from build123d import *

# Parameters (mm, degrees)
SKETCH1_W                   = 33
SKETCH1_H                   = 26
BOSS_EXTRUDE1_DEPTH         = 3.1
SKETCH3_W                   = 4
SKETCH3_H                   = 18
BOSS_EXTRUDE2_DEPTH         = 0.1
TAP_DRILL_FOR_M2X0_4_TAP2_D = 1.8
FILLET2_R                   = 1
SKETCH11_W                  = 21
SKETCH11_H                  = 14
CUT_EXTRUDE2_DEPTH          = 25.459005547


with BuildPart() as part:
    # Sketch1 → Boss-Extrude1 (new body)
    with BuildSketch(Plane(origin=(0, 0, 0), x_dir=(1, 0, 0), z_dir=(0, 1, 0))):
        with Locations((1.816045381, -2.910858995)):
            Rectangle(SKETCH1_W, SKETCH1_H)
    extrude(amount=BOSS_EXTRUDE1_DEPTH)

    # Sketch3 → Boss-Extrude2 (add)
    with BuildSketch(Plane(origin=(0, 3.1, 0), x_dir=(1, 0, 0), z_dir=(0, 1, 0))):
        Polygon((-10.683954619, 10.089141005), (-14.683954619, 10.089141005), (-14.683954619, -15.910858995), (-10.683954619, -15.910858995), (-10.683954619, -11.910858995), (-10.683954619, 6.089141005), align=None)
        Polygon((18.316045381, 10.089141005), (-10.683954619, 10.089141005), (-10.683954619, 6.089141005), (14.316045381, 6.089141005), (18.316045381, 6.089141005), align=None)
        Polygon((-10.683954619, -11.910858995), (-10.683954619, -15.910858995), (18.316045381, -15.910858995), (18.316045381, -11.910858995), (14.316045381, -11.910858995), align=None)
        with Locations((16.316045381, -2.910858995)):
            Rectangle(SKETCH3_W, SKETCH3_H)
    extrude(amount=BOSS_EXTRUDE2_DEPTH)

    # Tap Drill for M2x0.4 Tap2 (through all)
    with Locations(Plane(origin=(0, 3.2, 0), x_dir=(1, 0, 0), z_dir=(0, 1, 0))):
        with Locations((-12.683954619, 8.089141005), (-12.674525688, 2.589141005), (-12.764705981, -2.910858995), (-12.764705981, -8.410858995), (-12.764705981, -13.910858995), (-5.433954619, 8.089141005), (1.816045381, 8.089141005), (1.735294019, -13.910858995), (-5.514705981, -13.910858995), (9.066045381, 8.089141005), (16.316045381, 8.089141005), (16.316045381, 2.589141005), (16.316045381, -2.910858995), (16.316045381, -8.410858995), (16.316045381, -13.910858995), (8.985294019, -13.910858995)):
            Hole(TAP_DRILL_FOR_M2X0_4_TAP2_D / 2)

    # Fillet2
    fillet2_edges = [part.edges().sort_by_distance(p)[0] for p in [
        (-14.683954619, 1.6, -10.089141005),
        (18.316045381, 1.6, -10.089141005),
        (18.316045381, 1.6, 15.910858995),
        (-14.683954619, 1.6, 15.910858995),
    ]]
    fillet(fillet2_edges, radius=FILLET2_R)

    # Sketch11 → Cut-Extrude2 (cut, through all)
    with BuildSketch(Plane(origin=(0, 3.1, 0), x_dir=(1, 0, 0), z_dir=(0, 1, 0))):
        with Locations((1.816045381, -2.910858995)):
            Rectangle(SKETCH11_W, SKETCH11_H)
    extrude(amount=-CUT_EXTRUDE2_DEPTH, mode=Mode.SUBTRACT)


solid = part.part
Input: part model. Units: mm. Frame: model coordinates. A direction names the side the tool comes from. Coordinates: 2 decimals unless noted, no trailing zeros. Order: outer loops, then holes, each group sorted by start corner. A loop starts at its lowest first (then second) coordinate and runs counter-clockwise, first axis right, second up.
1. Ray query, line 1 along Z through (x, y) = (9, 1.35); line 2 along Z through (x, y) = (4.5, 2.4); line 3 along X through (y, z) = (1.3, 8.25). Return the intervals inside material, ascending.
Checked values:
line 1: z = -10.09 to -8.99, -7.19 to -4.09, 9.91 to 13.01, 14.81 to 15.91
line 2: z = -10.09 to -4.09, 9.91 to 15.91
line 3: x = -14.68 to -13.65, -11.88 to -8.68, 12.32 to 15.43, 17.2 to 18.32
2. Cut plane D-D, the plane z = 11.5. Return loops of the section in (x, y), plus the area to 3 significant figures.
Checked values:
outline: (-14.68, 0) - (18.32, 0) - (18.32, 3.2) - (14.32, 3.2) - (14.32, 3.1) - (-10.68, 3.1) - (-10.68, 3.2) - (-14.68, 3.2) - close
area: 103 mm2
3. Cut plane C-C, the plane x = -10. Return loops of the section in (y, z), plus the area to 3 significant figures.
Checked values:
outline: (0, -10.09) - (3.2, -10.09) - (3.2, -6.09) - (3.1, -6.09) - (3.1, 11.91) - (3.2, 11.91) - (3.2, 15.91) - (0, 15.91) - close
area: 81.4 mm2
4. Cut plane A-A, the plane x = -4. Return loops of the section in (y, z).
Checked values:
outline: (0, -10.09) - (3.2, -10.09) - (3.2, -6.09) - (3.1, -6.09) - (3.1, -4.09) - (0, -4.09) - close; (0, 9.91) - (3.1, 9.91) - (3.1, 11.91) - (3.2, 11.91) - (3.2, 15.91) - (0, 15.91) - close
5. Cut plane B-B, the plane z = -3. Return loops of the section in (x, y), plus the area to 3 significant figures.
Checked values:
outline: (-14.68, 0) - (-13.48, 0) - (-13.48, 3.2) - (-14.68, 3.2) - close; (-11.87, 0) - (-8.68, 0) - (-8.68, 3.1) - (-10.68, 3.1) - (-10.68, 3.2) - (-11.87, 3.2) - close; (12.32, 0) - (15.52, 0) - (15.52, 3.2) - (14.32, 3.2) - (14.32, 3.1) - (12.32, 3.1) - close; (17.12, 0) - (18.32, 0) - (18.32, 3.2) - (17.12, 3.2) - close
area: 27.8 mm2
6. Draft query along X for faces 4 (the cylindrical face through (-13.623, 1.578, 8.141)), 5 (the flat face through (2, 2, 9.911)), 6 (the cylindrical face through (-14.4, 1.62, 15.61)), 7 (the cylindrical face through (18.015, 1.622, 15.626)). Return one class per face: +X half, -X half, draft (parallel to the pull), parting line (faces both ways), or undercut.
Checked values:
face 4: undercut
face 5: undercut
face 6: -X half
face 7: +X half
7. Access query for faces 1 (the flat face through (18.316, 2, 3)), 2 (the flat face through (12.316, 2, 3)), 3 (the flat face through (2, 3.1, 11)). Directions: +Z, -Z, +X, -X, +Y, -Y. A direction counts if a zero-diameter tool reaches every point of the face in a straight line with its end or side. Return the directions, or none.
Checked values:
face 1: +Z, -Z, +X, +Y, -Y
face 2: +Y, -Y
face 3: +Y
